```python
from build123d import *

# Parameters (mm, degrees)
SKETCH1_W            = 25.4
SKETCH1_H            = 25.4
BOSS_EXTRUDE1_DEPTH  = 56.75
SKETCH2_W            = 23.8125
SKETCH2_H            = 23.8125
CUT_EXTRUDE1_DEPTH   = 115.912270885
FILLET1_R            = 0.508
M3_CLEARANCE_HOLE1_D = 3.4
M3_CLEARANCE_HOLE2_D = 3.4
M3_CLEARANCE_HOLE3_D = 3.4
M3_CLEARANCE_HOLE4_D = 3.4
FILLET2_R            = 1
CUT_EXTRUDE2_REACH   = 65.459
SKETCH11_W           = 16.9
SKETCH11_H           = 6.499999954
SKETCH11_H_2         = 7
CUT_EXTRUDE3_REACH   = 65.459
SKETCH12_W           = 16.9
SKETCH12_H           = 6.5
SKETCH12_H_2         = 7
FILLET3_R            = 3.81
CUT_EXTRUDE4_REACH   = 65.459
SKETCH13_W           = 15.4
SKETCH13_H           = 87.3
CUT_EXTRUDE5_REACH   = 65.459
SKETCH14_W           = 15.4
SKETCH14_H           = 87.3
CHAMFER2_SIZE        = 6.35
FILLET5_R            = 3.81


with BuildPart() as part:
    # Sketch1 → Boss-Extrude1 (new, symmetric)
    with BuildSketch(Plane(origin=(0, 0, 0), x_dir=(1, 0, 0), z_dir=(0, 1, 0))):
        Rectangle(SKETCH1_W, SKETCH1_H)
    extrude(amount=BOSS_EXTRUDE1_DEPTH, both=True)

    # Sketch2 → Cut-Extrude1 (cut, through all)
    with BuildSketch(Plane(origin=(0, 56.75, 0), x_dir=(1, 0, 0), z_dir=(0, 1, 0))):
        with Locations((0.79375, 0.79375)):
            Rectangle(SKETCH2_W, SKETCH2_H)
    extrude(amount=-CUT_EXTRUDE1_DEPTH, mode=Mode.SUBTRACT)

    # Fillet1
    fillet1_edges = [part.edges().sort_by_distance(p)[0] for p in [
        (-11.1125, 0, 11.1125),
    ]]
    fillet(fillet1_edges, radius=FILLET1_R)

    # M3 Clearance Hole1 (through all)
    with Locations(Plane.XY.offset(12.7)):
        with Locations((6.35, 47.075)):
            Hole(M3_CLEARANCE_HOLE1_D / 2)

    # M3 Clearance Hole2 (through all)
    with Locations(Plane.ZY.offset(12.7)):
        with Locations((-6.35, 47.075)):
            Hole(M3_CLEARANCE_HOLE2_D / 2)

    # M3 Clearance Hole3 (through all)
    with Locations(Plane.XY.offset(12.7)):
        with Locations((6.35, -46.575)):
            Hole(M3_CLEARANCE_HOLE3_D / 2)

    # M3 Clearance Hole4 (through all)
    with Locations(Plane.ZY.offset(12.7)):
        with Locations((-6.35, -46.575)):
            Hole(M3_CLEARANCE_HOLE4_D / 2)

    # Fillet2
    fillet2_edges = [part.edges().sort_by_distance(p)[0] for p in [
        (-12.7, 0, 12.7),
    ]]
    fillet(fillet2_edges, radius=FILLET2_R)

    # Sketch11 → Cut-Extrude2 (cut, up to next)
    with BuildSketch(Plane.ZY.offset(12.7), mode=Mode.PRIVATE) as cut_extrude2_sk1:
        with Locations((-4.25, 53.500000023)):
            Rectangle(SKETCH11_W, SKETCH11_H)
    cut_extrude2_tool1 = extrude(cut_extrude2_sk1.sketch, amount=-CUT_EXTRUDE2_REACH, mode=Mode.PRIVATE) & part.part
    # Sketch11 → Cut-Extrude2 (cut, up to next)
    with BuildSketch(Plane.ZY.offset(12.7), mode=Mode.PRIVATE) as cut_extrude2_sk2:
        with Locations((-4.25, -53.25)):
            Rectangle(SKETCH11_W, SKETCH11_H_2)
    cut_extrude2_tool2 = extrude(cut_extrude2_sk2.sketch, amount=-CUT_EXTRUDE2_REACH, mode=Mode.PRIVATE) & part.part
    add(cut_extrude2_tool1.solids().sort_by_distance((-12.7, 53.5, -4.25))[0], mode=Mode.SUBTRACT)
    add(cut_extrude2_tool2.solids().sort_by_distance((-12.7, -53.25, -4.25))[0], mode=Mode.SUBTRACT)

    # Sketch12 → Cut-Extrude3 (cut, up to next)
    with BuildSketch(Plane.XY.offset(12.7), mode=Mode.PRIVATE) as cut_extrude3_sk1:
        with Locations((4.25, 53.5)):
            Rectangle(SKETCH12_W, SKETCH12_H)
    cut_extrude3_tool1 = extrude(cut_extrude3_sk1.sketch, amount=-CUT_EXTRUDE3_REACH, mode=Mode.PRIVATE) & part.part
    # Sketch12 → Cut-Extrude3 (cut, up to next)
    with BuildSketch(Plane.XY.offset(12.7), mode=Mode.PRIVATE) as cut_extrude3_sk2:
        with Locations((4.25, -53.25)):
            Rectangle(SKETCH12_W, SKETCH12_H_2)
    cut_extrude3_tool2 = extrude(cut_extrude3_sk2.sketch, amount=-CUT_EXTRUDE3_REACH, mode=Mode.PRIVATE) & part.part
    add(cut_extrude3_tool1.solids().sort_by_distance((4.25, 53.5, 12.7))[0], mode=Mode.SUBTRACT)
    add(cut_extrude3_tool2.solids().sort_by_distance((4.25, -53.25, 12.7))[0], mode=Mode.SUBTRACT)

    # Fillet3
    fillet3_edges = [part.edges().sort_by_distance(p)[0] for p in [
        (-4.2, 50.25, 11.90625),
        (-4.2, -49.75, 11.90625),
        (-11.90625, 50.250000046, 4.2),
        (-11.90625, -49.75, 4.2),
    ]]
    fillet(fillet3_edges, radius=FILLET3_R)

    # Sketch13 → Cut-Extrude4 (cut, up to next)
    with BuildSketch(Plane.ZY.offset(12.7), mode=Mode.PRIVATE) as cut_extrude4_sk1:
        with Locations((-5, 0.25)):
            Rectangle(SKETCH13_W, SKETCH13_H)
    cut_extrude4_tool1 = extrude(cut_extrude4_sk1.sketch, amount=-CUT_EXTRUDE4_REACH, mode=Mode.PRIVATE) & part.part
    add(cut_extrude4_tool1.solids().sort_by_distance((-12.7, 0.25, -5))[0], mode=Mode.SUBTRACT)

    # Sketch14 → Cut-Extrude5 (cut, up to next)
    with BuildSketch(Plane.XY.offset(12.7), mode=Mode.PRIVATE) as cut_extrude5_sk1:
        with Locations((5, 0.25)):
            Rectangle(SKETCH14_W, SKETCH14_H)
    cut_extrude5_tool1 = extrude(cut_extrude5_sk1.sketch, amount=-CUT_EXTRUDE5_REACH, mode=Mode.PRIVATE) & part.part
    add(cut_extrude5_tool1.solids().sort_by_distance((5, 0.25, 12.7))[0], mode=Mode.SUBTRACT)

    # Chamfer2
    chamfer2_edges = [part.edges().sort_by_distance(p)[0] for p in [
        (-11.90625, 43.9, 2.7),
        (-11.90625, -43.4, 2.7),
        (-2.7, -43.4, 11.90625),
        (-2.7, 43.9, 11.90625),
    ]]
    chamfer(chamfer2_edges, length=CHAMFER2_SIZE)

    # Fillet5
    fillet5_edges = [part.edges().sort_by_distance(p)[0] for p in [
        (-11.90625, 43.9, -3.65),
        (-11.90625, -37.05, 2.7),
        (-11.90625, 37.55, 2.7),
        (-2.7, -37.05, 11.90625),
        (-2.7, 37.55, 11.90625),
        (3.65, 43.9, 11.90625),
        (3.65, -43.4, 11.90625),
        (-11.90625, -43.4, -3.65),
    ]]
    fillet(fillet5_edges, radius=FILLET5_R)


solid = part.part
```
The listing builds one solid part. Answer for the finished solid, in the listing's coordinates (mm). A direction names the side the tool comes from. Coordinates: 2 decimals unless noted, no trailing zeros. Loops run counter-clockwise (first coordinate to the right, second up) from the corner with the lowest first, then second, coordinate; pieces in that order, holes last. Notation, with made-up numbers: (52.5, 67.25) - (84.5, 67.25) arc R28 cw to (84.5, 102.25) - close; hole circle Ø3 at (-31.5, 52.5). An arc over 180 degrees is marked (long way). Use a Markdown table: item, result. Add a question column.
1) The part is cut by section B-B, the plane z = -6.35. State how many separate pieces and enclosed holes the cut face has, and give its area (3 significant figures).
2) Given pin 1 (1.3 mm diameter, centred on x = -12, y = -6.5, fed in from -Z); pin 2 (0.5 mm diameter, centred on x = 7, z = 12, fed in from +Y); pin 3 (1.3 mm diameter, centred on x = -12, z = -9, fed in from -Y), each flat-ended and moving along its own axis, determine where each tip first touches the part or whether it passes through.
3) Find the intervals of material crossed by line 1 (Y direction, x = -12.1, z = -6.35) (3 decimals); line 2 (Z direction, x = -9, y = 11), in increasing order.
4) The part is cut by section A-A, the plane x = 1.5. Give the vertices of the cut face in (y, z), and give its area (3 significant figures).
5) For faces 5 (the flat face through (-11.112, -12, 4)), 6 (the flat face through (0.45, 40.7, 11.92)), 7 (the flat face through (-11.92, 40.7, -0.45)), determine the directions among +Z, -Z, +X, -X, +Y, -Y from which every point of the face is accessible in a straight line to the end or side of a thin tool.
6) The part is cut by section C-C, the plane y = 1. Give the vertices of the cut face in (x, z).
7) The mould has two halves that part along Z. Classify faces 1 (the cylindrical face through (-3.114, -50.896, 11.895)), 2 (the cylindrical face through (-11.895, 45.415, -5.981)), 3 (the flat face through (-5, -12, 12.7)), 4 (the cylindrical face through (-11.895, 51.396, 3.114)): released by +Z, released by -Z, zero draft, split by the parting line, or undercut.
Here are the results:
| question | item | result |
|---|---|---|
| 1 | separate pieces | 4 |
| 1 | enclosed holes | 0 |
| 1 | area | 9.37 mm^2 |
| 2 | pin 1 | stops at z = 2.7 |
| 2 | pin 2 | stops at y = 50.25 |
| 2 | pin 3 | stops at y = -49.75 |
| 3 | line 1 | y = -49.75 to -48.275, -44.875 to -43.4, 43.9 to 45.375, 48.775 to 50.25 |
| 3 | line 2 | z = 11.11 to 12.7 |
| 4 | outline | (-49.75, 11.11) - (-41.25, 11.11) - (-41.25, 12.7) - (-49.75, 12.7) - close; (41.75, 11.11) - (50.25, 11.11) - (50.25, 12.7) - (41.75, 12.7) - close |
| 4 | area | 27.0 mm^2 |
| 5 | face 5 | -Z, +X, +Y, -Y |
| 5 | face 6 | +Z, -Z, +X |
| 5 | face 7 | -Z, +X, -X |
| 6 | outline | (-12.7, 2.7) - (-11.11, 2.7) - (-11.11, 10.6) arc R0.51 cw to (-10.6, 11.11) - (-2.7, 11.11) - (-2.7, 12.7) - (-11.7, 12.7) arc R1 ccw to (-12.7, 11.7) - close |
| 7 | face 1 | zero draft |
| 7 | face 2 | undercut |
| 7 | face 3 | released by +Z |
| 7 | face 4 | released by -Z |
